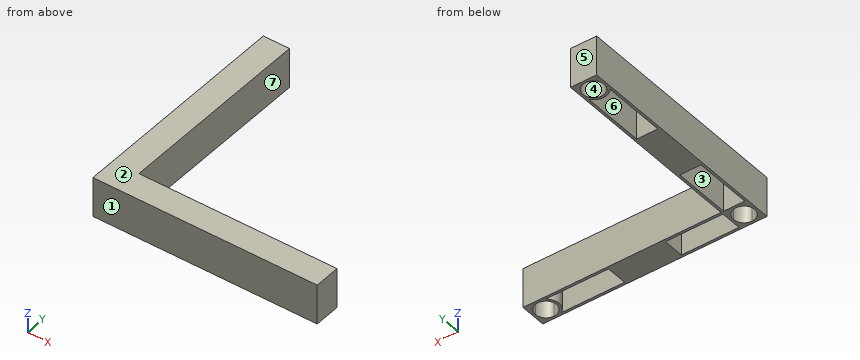
```python
from build123d import *

# Parameters (mm, degrees)
F0_W     = 16.1
F0_H     = 6
F0_W_2   = 6
F0_H_2   = 16.1
F0_W_3   = 0.7
F0_H_3   = 0.7
F1_DEPTH = 11.3
F2_DEPTH = 6
F3_DEPTH = 10


with BuildPart() as f1:
    # F0 (on Top) → F1 (new body)
    with BuildSketch(Plane.XY):
        with BuildLine():
            ThreePointArc((59.8, 6.7), (56.8, 3.7), (59.8, 0.7))
            ThreePointArc((59.8, 0.7), (61.9213203436, 1.5786796564), (62.8, 3.7))
            ThreePointArc((62.8, 3.7), (61.9213203436, 5.8213203436), (59.8, 6.7))
        make_face()
        with BuildLine():
            Line((7.4, 0.7), (7.4, 0))
            Line((7.4, 0), (59.8, 0))
            ThreePointArc((59.8, 0), (58.6620193323, 0.1793466515), (57.6343592172, 0.7))
            Line((57.6343592172, 0.7), (39.8, 0.7))
            Line((39.8, 0.7), (23.7, 0.7))
            Line((23.7, 0.7), (7.4, 0.7))
        make_face()
        with BuildLine():
            Line((3.7, 0.7), (5.8656407828, 0.7))
            ThreePointArc((5.8656407828, 0.7), (6.9941517039, 2.0151959901), (7.4, 3.7))
            ThreePointArc((7.4, 3.7), (7.2206533485, 4.8379806677), (6.7, 5.8656407828))
            Line((6.7, 5.8656407828), (6.7, 3.7))
            ThreePointArc((6.7, 3.7), (5.8213203436, 1.5786796564), (3.7, 0.7))
        make_face()
        with BuildLine():
            Line((0.7, 59.8), (0.7, 57.6343592172))
            ThreePointArc((0.7, 57.6343592172), (3.7, 56.1), (6.7, 57.6343592172))
            Line((6.7, 57.6343592172), (6.7, 59.8))
            ThreePointArc((6.7, 59.8), (3.7, 56.8), (0.7, 59.8))
        make_face()
        Polygon((0.7, 23.7), (0.7, 7.4), (3.7, 7.4), (6.7, 7.4), (6.7, 23.7), align=None)
        with BuildLine():
            Line((39.8, 0.7), (57.6343592172, 0.7))
            ThreePointArc((57.6343592172, 0.7), (56.1, 3.7), (57.6343592172, 6.7))
            Line((57.6343592172, 6.7), (39.8, 6.7))
            Line((39.8, 6.7), (39.8, 0.7))
        make_face()
        with BuildLine():
            ThreePointArc((3.7, 6.7), (5.8213203436, 5.8213203436), (6.7, 3.7))
            Line((6.7, 3.7), (6.7, 5.8656407828))
            ThreePointArc((6.7, 5.8656407828), (6.3162950904, 6.3162950904), (5.8656407828, 6.7))
            Line((5.8656407828, 6.7), (3.7, 6.7))
        make_face()
        with BuildLine():
            Line((6.7, 23.7), (6.7, 7.4))
            Line((6.7, 7.4), (7.4, 7.4))
            Line((7.4, 7.4), (7.4, 59.8))
            ThreePointArc((7.4, 59.8), (7.2206533485, 58.6620193323), (6.7, 57.6343592172))
            Line((6.7, 57.6343592172), (6.7, 39.8))
            Line((6.7, 39.8), (6.7, 23.7))
        make_face()
        with BuildLine():
            ThreePointArc((57.6343592172, 0.7), (58.6620193323, 0.1793466515), (59.8, 0))
            ThreePointArc((59.8, 0), (62.4162950904, 1.0837049096), (63.5, 3.7))
            ThreePointArc((63.5, 3.7), (62.4162950904, 6.3162950904), (59.8, 7.4))
            ThreePointArc((59.8, 7.4), (58.6620193323, 7.2206533485), (57.6343592172, 6.7))
            Line((57.6343592172, 6.7), (59.8, 6.7))
            ThreePointArc((59.8, 6.7), (61.9213203436, 5.8213203436), (62.8, 3.7))
            ThreePointArc((62.8, 3.7), (61.9213203436, 1.5786796564), (59.8, 0.7))
            Line((59.8, 0.7), (57.6343592172, 0.7))
        make_face()
        with BuildLine():
            Line((0, 63.5), (0, 59.8))
            ThreePointArc((0, 59.8), (1.0837049096, 62.4162950904), (3.7, 63.5))
            Line((3.7, 63.5), (0, 63.5))
        make_face()
        with BuildLine():
            ThreePointArc((63.5, 3.7), (62.4162950904, 1.0837049096), (59.8, 0))
            Line((59.8, 0), (63.5, 0))
            Line((63.5, 0), (63.5, 3.7))
        make_face()
        with BuildLine():
            Line((7.4, 63.5), (3.7, 63.5))
            ThreePointArc((3.7, 63.5), (6.3162950904, 62.4162950904), (7.4, 59.8))
            Line((7.4, 59.8), (7.4, 63.5))
        make_face()
        with BuildLine():
            ThreePointArc((59.8, 7.4), (62.4162950904, 6.3162950904), (63.5, 3.7))
            Line((63.5, 3.7), (63.5, 7.4))
            Line((63.5, 7.4), (59.8, 7.4))
        make_face()
        with BuildLine():
            Line((0, 59.8), (0, 7.4))
            Line((0, 7.4), (0.7, 7.4))
            Line((0.7, 7.4), (0.7, 23.7))
            Line((0.7, 23.7), (0.7, 39.8))
            Line((0.7, 39.8), (0.7, 57.6343592172))
            ThreePointArc((0.7, 57.6343592172), (0.1793466515, 58.6620193323), (0, 59.8))
        make_face()
        with BuildLine():
            ThreePointArc((57.6343592172, 6.7), (56.1, 3.7), (57.6343592172, 0.7))
            Line((57.6343592172, 0.7), (59.8, 0.7))
            ThreePointArc((59.8, 0.7), (56.8, 3.7), (59.8, 6.7))
            Line((59.8, 6.7), (57.6343592172, 6.7))
        make_face()
        with BuildLine():
            ThreePointArc((6.7, 57.6343592172), (3.7, 56.1), (0.7, 57.6343592172))
            Line((0.7, 57.6343592172), (0.7, 39.8))
            Line((0.7, 39.8), (6.7, 39.8))
            Line((6.7, 39.8), (6.7, 57.6343592172))
        make_face()
        Polygon((7.4, 3.7), (7.4, 0.7), (23.7, 0.7), (23.7, 6.7), (7.4, 6.7), align=None)
        with BuildLine():
            ThreePointArc((3.7, 7.4), (2.0151959901, 6.9941517039), (0.7, 5.8656407828))
            Line((0.7, 5.8656407828), (0.7, 3.7))
            ThreePointArc((0.7, 3.7), (1.5786796564, 5.8213203436), (3.7, 6.7))
            Line((3.7, 6.7), (5.8656407828, 6.7))
            ThreePointArc((5.8656407828, 6.7), (4.8379806677, 7.2206533485), (3.7, 7.4))
        make_face()
        with Locations((31.75, 3.7)):
            Rectangle(F0_W, F0_H)
        with BuildLine():
            ThreePointArc((6.7, 59.8), (3.7, 62.8), (0.7, 59.8))
            ThreePointArc((0.7, 59.8), (3.7, 56.8), (6.7, 59.8))
        make_face()
        with BuildLine():
            ThreePointArc((0, 3.7000000003), (1.0837049095, 1.0837049097), (3.7, 0))
            ThreePointArc((3.7, 0), (4.8379806677, 0.1793466515), (5.8656407828, 0.7))
            Line((5.8656407828, 0.7), (3.7, 0.7))
            ThreePointArc((3.7, 0.7), (1.5786796564, 1.5786796564), (0.7, 3.7))
            Line((0.7, 3.7), (0.7, 5.8656407828))
            ThreePointArc((0.7, 5.8656407828), (0.1793466516, 4.8379806678), (0, 3.7000000003))
        make_face()
        with BuildLine():
            ThreePointArc((3.7, 63.5), (1.0837049096, 62.4162950904), (0, 59.8))
            ThreePointArc((0, 59.8), (0.1793466515, 58.6620193323), (0.7, 57.6343592172))
            Line((0.7, 57.6343592172), (0.7, 59.8))
            ThreePointArc((0.7, 59.8), (3.7, 62.8), (6.7, 59.8))
            Line((6.7, 59.8), (6.7, 57.6343592172))
            ThreePointArc((6.7, 57.6343592172), (7.2206533485, 58.6620193323), (7.4, 59.8))
            ThreePointArc((7.4, 59.8), (6.3162950904, 62.4162950904), (3.7, 63.5))
        make_face()
        with Locations((3.7, 31.75)):
            Rectangle(F0_W_2, F0_H_2)
        with BuildLine():
            ThreePointArc((0.7, 3.7), (1.5786796564, 1.5786796564), (3.7, 0.7))
            ThreePointArc((3.7, 0.7), (5.8213203436, 1.5786796564), (6.7, 3.7))
            ThreePointArc((6.7, 3.7), (5.8213203436, 5.8213203436), (3.7, 6.7))
            ThreePointArc((3.7, 6.7), (1.5786796564, 5.8213203436), (0.7, 3.7))
        make_face()
        with BuildLine():
            Line((0, 3.7000000003), (0, 0))
            Line((0, 0), (3.7, 0))
            ThreePointArc((3.7, 0), (1.0837049095, 1.0837049097), (0, 3.7000000003))
        make_face()
        with BuildLine():
            ThreePointArc((5.8656407828, 6.7), (6.3162950904, 6.3162950904), (6.7, 5.8656407828))
            Line((6.7, 5.8656407828), (6.7, 6.7))
            Line((6.7, 6.7), (5.8656407828, 6.7))
        make_face()
        with BuildLine():
            Line((7.4, 7.4), (7.4, 6.7))
            Line((7.4, 6.7), (23.7, 6.7))
            Line((23.7, 6.7), (39.8, 6.7))
            Line((39.8, 6.7), (57.6343592172, 6.7))
            ThreePointArc((57.6343592172, 6.7), (58.6620193323, 7.2206533485), (59.8, 7.4))
            Line((59.8, 7.4), (7.4, 7.4))
        make_face()
        with BuildLine():
            ThreePointArc((5.8656407828, 0.7), (4.8379806677, 0.1793466515), (3.7, 0))
            Line((3.7, 0), (7.4, 0))
            Line((7.4, 0), (7.4, 0.7))
            Line((7.4, 0.7), (5.8656407828, 0.7))
        make_face()
        with BuildLine():
            Line((0.7, 7.4), (0.7, 5.8656407828))
            ThreePointArc((0.7, 5.8656407828), (2.0151959901, 6.9941517039), (3.7, 7.4))
            Line((3.7, 7.4), (0.7, 7.4))
        make_face()
        with BuildLine():
            Line((0, 7.4), (0, 3.7000000003))
            ThreePointArc((0, 3.7000000003), (0.1793466516, 4.8379806678), (0.7, 5.8656407828))
            Line((0.7, 5.8656407828), (0.7, 7.4))
            Line((0.7, 7.4), (0, 7.4))
        make_face()
        with BuildLine():
            Line((6.7, 7.4), (3.7, 7.4))
            ThreePointArc((3.7, 7.4), (4.8379806677, 7.2206533485), (5.8656407828, 6.7))
            Line((5.8656407828, 6.7), (6.7, 6.7))
            Line((6.7, 6.7), (6.7, 7.4))
        make_face()
        with BuildLine():
            ThreePointArc((7.4, 3.7), (6.9941517039, 2.0151959901), (5.8656407828, 0.7))
            Line((5.8656407828, 0.7), (7.4, 0.7))
            Line((7.4, 0.7), (7.4, 3.7))
        make_face()
        with BuildLine():
            ThreePointArc((6.7, 5.8656407828), (7.2206533485, 4.8379806677), (7.4, 3.7))
            Line((7.4, 3.7), (7.4, 6.7))
            Line((7.4, 6.7), (6.7, 6.7))
            Line((6.7, 6.7), (6.7, 5.8656407828))
        make_face()
        with Locations((7.05, 7.05)):
            Rectangle(F0_W_3, F0_H_3)
    extrude(amount=F1_DEPTH)

    # F0 (on Top) → F2 (cut)
    with BuildSketch(Plane.XY):
        with BuildLine():
            ThreePointArc((6.7, 59.8), (3.7, 62.8), (0.7, 59.8))
            ThreePointArc((0.7, 59.8), (3.7, 56.8), (6.7, 59.8))
        make_face()
        with BuildLine():
            ThreePointArc((0.7, 3.7), (1.5786796564, 1.5786796564), (3.7, 0.7))
            ThreePointArc((3.7, 0.7), (5.8213203436, 1.5786796564), (6.7, 3.7))
            ThreePointArc((6.7, 3.7), (5.8213203436, 5.8213203436), (3.7, 6.7))
            ThreePointArc((3.7, 6.7), (1.5786796564, 5.8213203436), (0.7, 3.7))
        make_face()
        with BuildLine():
            ThreePointArc((59.8, 6.7), (56.8, 3.7), (59.8, 0.7))
            ThreePointArc((59.8, 0.7), (61.9213203436, 1.5786796564), (62.8, 3.7))
            ThreePointArc((62.8, 3.7), (61.9213203436, 5.8213203436), (59.8, 6.7))
        make_face()
    extrude(amount=F2_DEPTH, mode=Mode.SUBTRACT)

    # F0 (on Top) → F3 (cut)
    with BuildSketch(Plane.XY):
        with BuildLine():
            ThreePointArc((6.7, 57.6343592172), (3.7, 56.1), (0.7, 57.6343592172))
            Line((0.7, 57.6343592172), (0.7, 39.8))
            Line((0.7, 39.8), (6.7, 39.8))
            Line((6.7, 39.8), (6.7, 57.6343592172))
        make_face()
        Polygon((0.7, 23.7), (0.7, 7.4), (3.7, 7.4), (6.7, 7.4), (6.7, 23.7), align=None)
        with BuildLine():
            Line((39.8, 0.7), (57.6343592172, 0.7))
            ThreePointArc((57.6343592172, 0.7), (56.1, 3.7), (57.6343592172, 6.7))
            Line((57.6343592172, 6.7), (39.8, 6.7))
            Line((39.8, 6.7), (39.8, 0.7))
        make_face()
        Polygon((7.4, 3.7), (7.4, 0.7), (23.7, 0.7), (23.7, 6.7), (7.4, 6.7), align=None)
    extrude(amount=F3_DEPTH, mode=Mode.SUBTRACT)


solid = f1.part
```
Geometry check sheet. Reference: the model listing, model coordinates, mm. Face numbers are marked on the shaded views. A direction names the side the tool comes from. Round coordinates to 2 decimals unless told otherwise and drop trailing zeros. Loops run counter-clockwise (first coordinate to the right, second up) from the corner with the lowest first, then second, coordinate; pieces in that order, holes last. Notation, with made-up numbers: (-33, 61.25) -> (-21, 61.25) arc R14 cw to (-21, 88.25) -> close; hole circle Ø5 at (85.5, 33). An arc over 180 degrees is marked (long way). Use a Markdown table: item, result.
(1) Scan lines: probe 1 along X at (y, z) = (14, 7.5); probe 2 along Y at (x, z) = (3, 9.25). Record each from-to range of solid material in increasing order.
Calculated:
| item | result |
|---|---|
| probe 1 | 0 to 0.7, 6.7 to 7.4 |
| probe 2 | 0 to 7.4, 23.7 to 39.8, 56.17 to 63.5 |
(2) Go/stop test with flat-tipped pins: P1, Ø4, axis at y = 27, z = 5.5, coming from the +X side; P2, Ø5, axis at x = 47.5, z = 5, coming from the +Y side; P3, Ø1.8, axis at x = 61, y = 3, coming from the -Z side. Record where each tip stops, or that it passes through.
Calculated:
| item | result |
|---|---|
| P1 | x = 7.4 |
| P2 | y = 7.4 |
| P3 | z = 6 |
(3) Sectioned sample at C-C (z = 1.5). Enter the section's corners in (x, y).
Calculated:
| item | result |
|---|---|
| outline | (0, 0) -> (63.5, 0) -> (63.5, 7.4) -> (7.4, 7.4) -> (7.4, 63.5) -> (0, 63.5) -> close; hole circle Ø6 at (3.7, 3.7); hole (0.7, 7.4) -> (6.7, 7.4) -> (6.7, 23.7) -> (0.7, 23.7) -> close; hole (0.7, 39.8) -> (6.7, 39.8) -> (6.7, 57.63) arc R3.7 cw to (0.7, 57.63) -> close; hole circle Ø6 at (3.7, 59.8); hole (7.4, 0.7) -> (23.7, 0.7) -> (23.7, 6.7) -> (7.4, 6.7) -> close; hole (39.8, 0.7) -> (57.63, 0.7) arc R3.7 cw to (57.63, 6.7) -> (39.8, 6.7) -> close; hole circle Ø6 at (59.8, 3.7) |
(4) Set-up check for the marked faces 5, 6 and 7: record each of +Z, -Z, +X, -X, +Y, -Y from which the full face is reachable in a straight line by a thin tool's end or side.
Calculated:
| item | result |
|---|---|
| face 5 | +Z, -Z, +X, -X, +Y |
| face 6 | -Z |
| face 7 | +Z, -Z, +X, +Y |
(5) Sectioned sample at A-A (x = 16.5). Enter the section's corners in (y, z), then the cut area to 3 significant figures.
Calculated:
| item | result |
|---|---|
| outline | (0, 0) -> (0.7, 0) -> (0.7, 10) -> (6.7, 10) -> (6.7, 0) -> (7.4, 0) -> (7.4, 11.3) -> (0, 11.3) -> close |
| area | 23.6 mm² |
(6) Mould release check, pull along Y, two halves, no side actions. Record for the marked faces 1, 2, 3 and 4: released by +Y, released by -Y, zero draft, split by the parting line, or undercut.
Calculated:
| item | result |
|---|---|
| face 1 | released by -Y |
| face 2 | zero draft |
| face 3 | undercut |
| face 4 | undercut |
(7) Sectioned sample at D-D (y = 4.5). Enter the section's corners in (x, z).
Calculated:
| item | result |
|---|---|
| outline | (0, 0) -> (0.81, 0) -> (0.81, 6) -> (6.59, 6) -> (6.59, 0) -> (7.4, 0) -> (7.4, 10) -> (23.7, 10) -> (23.7, 0) -> (39.8, 0) -> (39.8, 10) -> (56.19, 10) -> (56.19, 0) -> (56.91, 0) -> (56.91, 6) -> (62.69, 6) -> (62.69, 0) -> (63.5, 0) -> (63.5, 11.3) -> (0, 11.3) -> close |
